```python
from build123d import *

# Parameters (mm, degrees)
BOSS_EXTRUDE1_DEPTH     = 6
BOSS_EXTRUDE2_DEPTH     = 10
BOSS_EXTRUDE3_DEPTH     = 6
SKETCH4_R               = 3
CUT_EXTRUDE1_DEPTH      = 41.311288741
TAP_DRILL_FOR_M3_TAP1_D = 2.5
TAP_DRILL_FOR_M3_TAP2_D = 2.5
CHAMFER1_SIZE           = 2
FILLET1_R               = 3
FILLET2_R               = 10
FILLET3_R               = 2


with BuildPart() as part:
    # Sketch1 → Boss-Extrude1 (new body)
    with BuildSketch(Plane.XY):
        with BuildLine():
            Line((20, 0), (25, 0))
            ThreePointArc((25, 0), (0, 25), (-25, 0))
            Line((-25, 0), (-20, 0))
            ThreePointArc((-20, 0), (0, 20), (20, 0))
        make_face()
    extrude(amount=BOSS_EXTRUDE1_DEPTH)

    # Sketch2 → Boss-Extrude2 (add)
    with BuildSketch(Plane.XY.offset(6)):
        with BuildLine():
            ThreePointArc((-20, 0), (-17.320508076, 10), (-10, 17.320508076))
            Line((-10, 17.320508076), (-12.5, 21.650635095))
            ThreePointArc((-12.5, 21.650635095), (-21.650635095, 12.5), (-25, 0))
            Line((-25, 0), (-20, 0))
        make_face()
        with BuildLine():
            Line((12.5, 21.650635095), (10, 17.320508076))
            ThreePointArc((10, 17.320508076), (17.320508076, 10), (20, 0))
            Line((20, 0), (25, 0))
            ThreePointArc((25, 0), (21.650635095, 12.5), (12.5, 21.650635095))
        make_face()
    extrude(amount=BOSS_EXTRUDE2_DEPTH)

    # Sketch3 → Boss-Extrude3 (add)
    with BuildSketch(Plane(origin=(0, 0, 0), x_dir=(-1, 0, 0), z_dir=(0, 0, -1))):
        with BuildLine():
            Line((-25, 0), (-25, 30))
            Line((-25, 30), (25, 30))
            Line((25, 30), (25, 0))
            ThreePointArc((25, 0), (0, 25), (-25, 0))
        make_face()
    extrude(amount=-BOSS_EXTRUDE3_DEPTH)

    # Sketch4 → Cut-Extrude1 (cut, through all)
    with BuildSketch(Plane.XY.offset(6)):
        with Locations((13, 25)):
            Circle(SKETCH4_R)
        with Locations((-13, 25)):
            Circle(SKETCH4_R)
    extrude(amount=-CUT_EXTRUDE1_DEPTH, mode=Mode.SUBTRACT)

    # Tap Drill for M3 Tap1 (through all)
    with Locations(Plane(origin=(-17.67766953, 17.67766953, 0), x_dir=(0, 0, -1), z_dir=(-0.7071067811865488, 0.7071067811865464, 0))):
        with Locations((-11, 7.071067812)):
            Hole(TAP_DRILL_FOR_M3_TAP1_D / 2)

    # Tap Drill for M3 Tap2 (through all)
    with Locations(Plane(origin=(17.67766953, 17.67766953, 0), x_dir=(0, 0, -1), z_dir=(0.7071067811865488, 0.7071067811865464, 0))):
        with Locations((-11, 0)):
            Hole(TAP_DRILL_FOR_M3_TAP2_D / 2)

    # Chamfer1
    # the kernel refuses this chamfer: 2 mm, written as the material it takes off along each edge
    with BuildSketch(Plane(origin=(-25, 0, 21.143365976), x_dir=(1, 0, 0), z_dir=(0, 0, -1))) as chamfer1_piece_1:
        with BuildLine():
            Line((CHAMFER1_SIZE, 0), (0.074278418, -1.925721582))
            ThreePointArc((0.074278418, -1.925721582), (0.019638133, -0.990717402), (0, 0))
            Line((0, 0), (CHAMFER1_SIZE, 0))
        make_face()
    extrude(amount=15.143365976, mode=Mode.SUBTRACT)
    with BuildSketch(Plane(origin=(25, 0, 21.143365976), x_dir=(-1, 0, 0), z_dir=(0, 0, -1))) as chamfer1_piece_2:
        with BuildLine():
            Line((CHAMFER1_SIZE, 0), (0.074278418, 1.925721582))
            ThreePointArc((0.074278418, 1.925721582), (0.019638133, 0.990717402), (0, 0))
            Line((0, 0), (CHAMFER1_SIZE, 0))
        make_face()
    extrude(amount=15.143365976, mode=Mode.SUBTRACT)

    # Fillet1
    fillet1_edges = [part.edges().sort_by_distance(p)[0] for p in [
        (-12.5, 21.650635095, 11),
        (12.5, 21.650635095, 11),
        (20, 0, 8),
        (-20, 0, 8),
    ]]
    fillet(fillet1_edges, radius=FILLET1_R)

    # Fillet2
    fillet2_edges = [part.edges().sort_by_distance(p)[0] for p in [
        (-25, 30, 3),
        (25, 30, 3),
    ]]
    fillet(fillet2_edges, radius=FILLET2_R)

    # Fillet3
    fillet3_edges = [part.edges().sort_by_distance(p)[0] for p in [
        (25, 0, 3),
        (-25, 0, 3),
    ]]
    fillet(fillet3_edges, radius=FILLET3_R)


solid = part.part
```
The listing builds one solid part. Answer for the finished solid, in the listing's coordinates (mm). A direction names the side the tool comes from. Give positions to 0.01 mm unless a question says otherwise; leave off trailing zeros. Order: outer loops, then holes, each group sorted by start corner. A loop starts at its lowest first (then second) coordinate and runs counter-clockwise, first axis right, second up. Notation, with made-up numbers: (14, 59) -> (53, 59) arc R17 ccw to (53, 75) -> close; hole circle Ø11 at (-7, -25). An arc over 180 degrees is marked (long way). Answer as CSV lines item,"result". Start each with the question number.
Q1. A cutting plane is placed at C-C (y = 25). Determine the outline of the cut face in (x, z).
Q2. Which of the six approach directions +Z, -Z, +X, -X, +Y, -Y give full straight-line access (tool end or side, diameter ignored) to faces 1 (the cylindrical face through (20.848, 0.725, 8.112)), 2 (the cylindrical face through (12.88, 20.31, 11.07)), 3 (the flat face through (19, 10, 16)), 4 (the cylindrical face through (-21.944, 11.977, 13.152)), 5 (the flat face through (24, 1, 11))?
Q3. A cutting plane is placed at A-A (z = 14). Determine the outline of the cut face in (x, y).
Q4. Determine the mould class of faces 6 (the flat face through (0, 22, 0)), 7 (the flat face through (-10.442, 18.087, 10.93)), 8 (the flat face through (-24, 1, 11)), 9 (the cylindrical face through (22.083, 11.72, 10.93)) for opening direction X: pulls with the +X half, pulls with the -X half, needs draft (parallel to the pull), parting line crosses it, or undercut.
Q5. Given pin 1 (5 mm diameter, centred on x = 13, y = 25, fed in from +Z), flat-ended and moving along its own axis, determine where the tip first touches the part or whether it passes through.
Q6. A cutting plane is placed at D-D (z = 1). Determine the outline of the cut face in (x, y).
Q7. A cutting plane is placed at B-B (x = -13). Determine the outline of the cut face in (y, z), then the cut area to 3 significant figures.
Q8. Find the intervals of material crossed by L1, parallel to Z at x = 15.5, y = 15.5; L2, parallel to Y at x = -13, z = 2.85; L3, parallel to Y at x = -14.5, z = 2, in increasing order.
Results found:
1,outline,"(-23.66, 0) -> (-16, 0) -> (-16, 6) -> (-23.66, 6) -> close; (-10, 0) -> (10, 0) -> (10, 6) -> (-10, 6) -> close; (16, 0) -> (23.66, 0) -> (23.66, 6) -> (16, 6) -> close"
2,face 1,"+Z, -Z, -Y"
2,face 2,"+Z, +Y"
2,face 3,"+Z, +X, -X, +Y, -Y"
2,face 4,"+Z, -X, +Y"
2,face 5,"+Z, +X, -Y"
3,outline,"(-24.93, 1.93) -> (-23, 0) -> (-22.8, 0) arc R3 ccw to (-19.83, 2.61) arc R20 cw to (-10, 17.32) -> (-10.9, 18.87) arc R3 ccw to (-15.34, 19.74) arc R25 ccw to start; (10, 17.32) arc R20 cw to (19.83, 2.61) arc R3 ccw to (22.8, 0) -> (23, 0) -> (24.93, 1.93) arc R25 ccw to (15.34, 19.74) arc R3 ccw to (10.9, 18.87) -> close"
4,face 6,"needs draft"
4,face 7,"undercut"
4,face 8,"pulls with the -X half"
4,face 9,"pulls with the +X half"
5,pin 1,"through"
6,outline,"(-25, 2) arc R2 ccw to (-23, 0) -> (-22.8, 0) arc R3 ccw to (-19.83, 2.61) arc R20 cw to (19.83, 2.61) arc R3 ccw to (22.8, 0) -> (23, 0) arc R2 ccw to (25, 2) -> (25, 20) arc R10 ccw to (15, 30) -> (-15, 30) arc R10 ccw to (-25, 20) -> close; hole circle Ø6 at (-13, 25); hole circle Ø6 at (13, 25)"
7,outline,"(15.2, 0) -> (22, 0) -> (22, 6) -> (20.33, 6) -> (20.33, 16) -> (15.2, 16) -> close; (28, 0) -> (30, 0) -> (30, 6) -> (28, 6) -> close"
7,area,"104 mm2"
8,L1,"0 to 9.75, 12.25 to 16"
8,L2,"15.2 to 22, 28 to 30"
8,L3,"13.77 to 22.4, 27.6 to 30"
